```python
from build123d import *

# Parameters (mm, degrees)
ESQUISSE1_W             = 156
ESQUISSE1_H             = 96
BOSS_EXTRU_1_DEPTH      = 2
ESQUISSE2_W             = 156
ESQUISSE2_H             = 96
ESQUISSE2_W_2           = 152
ESQUISSE2_H_2           = 92
BOSS_EXTRU_2_DEPTH      = 18
ESQUISSE3_W             = 12
ESQUISSE3_H             = 12
BOSS_EXTRU_3_DEPTH      = 5
ESQUISSE4_W             = 12.488308145
ESQUISSE4_H             = 26
ESQUISSE4_W_2           = 11
ESQUISSE4_H_2           = 11.218310707
ENL_V_MAT_EXTRU_1_DEPTH = 100.689086297


with BuildPart() as part:
    # Esquisse1 → Boss.-Extru.1 (new body)
    with BuildSketch(Plane.XY):
        with Locations((7.861406509, -1.444239291)):
            Rectangle(ESQUISSE1_W, ESQUISSE1_H)
    extrude(amount=BOSS_EXTRU_1_DEPTH)

    # Esquisse2 → Boss.-Extru.2 (add)
    with BuildSketch(Plane.XY.offset(2)):
        with Locations((7.861406509, -1.444239291)):
            Rectangle(ESQUISSE2_W, ESQUISSE2_H)
        with Locations((7.861406509, -1.444239291)):
            Rectangle(ESQUISSE2_W_2, ESQUISSE2_H_2, mode=Mode.SUBTRACT)
    extrude(amount=BOSS_EXTRU_2_DEPTH)

    # Esquisse3 → Boss.-Extru.3 (add)
    with BuildSketch(Plane.XY.offset(2)):
        with Locations((-62.138593491, 38.555760709)):
            Rectangle(ESQUISSE3_W, ESQUISSE3_H)
        with Locations((77.861406509, -41.444239291)):
            Rectangle(ESQUISSE3_W, ESQUISSE3_H)
        with Locations((77.861406509, 38.555760709)):
            Rectangle(ESQUISSE3_W, ESQUISSE3_H)
        with Locations((-62.138593491, -41.444239291)):
            Rectangle(ESQUISSE3_W, ESQUISSE3_H)
    extrude(amount=BOSS_EXTRU_3_DEPTH)

    # Esquisse4 → Enlèv. mat.-Extru.1 (cut, through all)
    with BuildSketch(Plane.XY.offset(9)):
        with Locations((-68.655939158, -27.444239291)):
            Rectangle(ESQUISSE4_W, ESQUISSE4_H)
        with Locations((-27.638593491, -49.280809473)):
            Rectangle(ESQUISSE4_W_2, ESQUISSE4_H_2)
    extrude(amount=ENL_V_MAT_EXTRU_1_DEPTH, mode=Mode.SUBTRACT)


solid = part.part
```
Work out the finished part from the listing and answer in its coordinate system (mm). A direction names the side the tool comes from. Round coordinates to 2 decimals unless told otherwise and drop trailing zeros. Loops run counter-clockwise (first coordinate to the right, second up) from the corner with the lowest first, then second, coordinate; pieces in that order, holes last. Notation, with made-up numbers: (41, 26) -> (57, 26) arc R24 cw to (57, 41) -> close; hole circle Ø9 at (89.5, 77). An arc over 180 degrees is marked (long way). Write each question's results on one line, items separated by ' | '. Start each with the question number.
1. Find the intervals of material crossed by probe 1 along Y at (x, z) = (18, 11); probe 2 along X at (y, z) = (-5.5, 18.5); probe 3 along X at (y, z) = (-38, 2.5), in increasing order. Write a range as from..to.
2. A tool of negligible diameter and unlimited length cuts with its end or side. For faces 4 (the face through (85.861, -2, 10)), 5 (the face through (-68.139, -2, 11)), from which of +Z, -Z, +X, -X, +Y, -Y can it reach the whole face along a straight path? Write none if from no direction.
3. Section B-B (y = -12.5) is taken. Determine the outline of the cut face in (x, z), plus the area to 3 significant figures.
4. Section D-D (y = -42) is taken. Determine the outline of the cut face in (x, z).
5. Given pin 1 Ø12 at (x, y) = (-52, -31.5) entering from +Z; pin 2 Ø10 at (y, z) = (-28.5, 12.5) entering from -X; pin 3 Ø1 at (x, y) = (-29, -48.5) entering from +Z, each flat-ended and moving along its own axis, determine where each tip first touches the part or whether it passes through.
6. Section A-A (z = 18) is taken. Determine the outline of the cut face in (x, y).
7. For a pull along Y with two mould halves and no side action, classify faces 1 (the face through (-70.139, -2, 10)), 2 (the face through (7, -49.444, 10)), 3 (the face through (78, -41, 7)) as +Y half, -Y half, draft (parallel to the pull), parting line (faces both ways), or undercut.
8. Section C-C (x = -46.5) is taken. Determine the outline of the cut face in (y, z).
Evaluation:
1) probe 1: y = -49.44..-47.44, 44.56..46.56 | probe 2: x = -70.14..-68.14, 83.86..85.86 | probe 3: x = -70.14..-56.14, 71.86..85.86
2) face 4: +Z, -Z, +X, +Y, -Y | face 5: +Z
3) outline: (-70.14, 0) -> (85.86, 0) -> (85.86, 20) -> (83.86, 20) -> (83.86, 2) -> (-68.14, 2) -> (-68.14, 20) -> (-70.14, 20) -> close | area: 384 mm2
4) outline: (-70.14, 0) -> (85.86, 0) -> (85.86, 20) -> (83.86, 20) -> (83.86, 7) -> (71.86, 7) -> (71.86, 2) -> (-56.14, 2) -> (-56.14, 7) -> (-68.14, 7) -> (-68.14, 20) -> (-70.14, 20) -> close
5) pin 1: stops at z = 7 | pin 2: stops at x = -70.14 | pin 3: stops at z = 9
6) outline: (-70.14, -49.44) -> (-33.14, -49.44) -> (-33.14, -47.44) -> (-68.14, -47.44) -> (-68.14, -40.44) -> (-70.14, -40.44) -> close; (-70.14, -14.44) -> (-68.14, -14.44) -> (-68.14, 44.56) -> (83.86, 44.56) -> (83.86, -47.44) -> (-22.14, -47.44) -> (-22.14, -49.44) -> (85.86, -49.44) -> (85.86, 46.56) -> (-70.14, 46.56) -> close
7) face 1: draft | face 2: -Y half | face 3: undercut
8) outline: (-49.44, 0) -> (46.56, 0) -> (46.56, 20) -> (44.56, 20) -> (44.56, 2) -> (-47.44, 2) -> (-47.44, 20) -> (-49.44, 20) -> close
